Geometry: final body of the model. Coordinates: model frame, mm. Give positions to 0.01 mm unless a question says otherwise; leave off trailing zeros. Write each loop counter-clockwise with the first axis right and the second up, starting at its lowest first coordinate (ties: lowest second). Pieces come first, ordered by that corner, then holes.
from build123d import *

# Parameters (mm, degrees)
SPHERE001_ANGLE = 180
SPHERE_ANGLE    = 180


with BuildPart() as inner:
    # Sphere001 → Sphere001 (revolve)
    with BuildSketch(Plane.XZ):
        with BuildLine():
            ThreePointArc((0, -28), (28, 0), (0, 28))
            Line((0, 28), (0, -28))
        make_face()
    revolve(axis=Axis((0, 0, 0), (0, 0, 1)), revolution_arc=SPHERE001_ANGLE)


with BuildPart() as cut:
    # Sphere → Sphere (revolve)
    with BuildSketch(Plane.XZ):
        with BuildLine():
            ThreePointArc((0, -30), (30, 0), (0, 30))
            Line((0, 30), (0, -30))
        make_face()
    revolve(axis=Axis((0, 0, 0), (0, 0, 1)), revolution_arc=SPHERE_ANGLE)

    # Cut: cut Inner
    add(inner.part, mode=Mode.SUBTRACT)


solid = cut.part
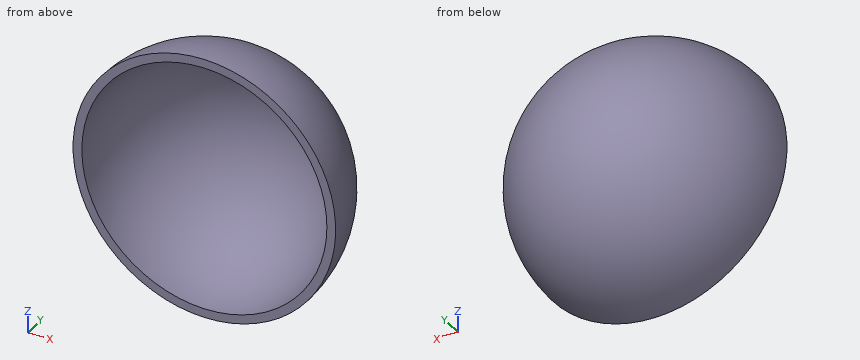
Q1. Section B-B on z = -1. Output: boundary loops of the cut face in (x, y).
Filled sheet:
outline: (-29.98, 0) - (-27.98, 0) arc R27.98 cw to (27.98, 0) - (29.98, 0) arc R29.98 ccw to start
Q2. Section C-C on x = 14. Output: boundary loops of the cut face in (y, z), plus the area to 3 significant figures.
Filled sheet:
outline: (0, -26.53) arc R26.53 ccw to (0, 26.53) - (0, 24.25) arc R24.25 cw to (0, -24.25) - close
area: 182 mm2
Q3. Pin query (flat end, axial travel): P1, Ø1.5, axis at x = 0, y = 8, coming from the -Z side; P2, Ø5, axis at x = -5, y = 25, coming from the +Z side; P3, Ø3, axis at y = 25.5, z = 1.5, coming from the +X side. Return the tip coordinate at first contact, or that it passes through.
Filled sheet:
P1: stops at z = -29.11
P2: stops at z = 19.27
P3: stops at x = 17.94
Q4. Ray query, line 1 along X through (y, z) = (10.5, -23); line 2 along Z through (x, y) = (12.5, 6.25); line 3 along X through (y, z) = (14.5, -8.5). Return the intervals inside material, ascending.
Filled sheet:
line 1: x = -16.15 to -12.03, 12.03 to 16.15
line 2: z = -26.55 to -24.26, 24.26 to 26.55
line 3: x = -24.85 to -22.39, 22.39 to 24.85
Q5. Section A-A on y = 16.25. Output: boundary loops of the cut face in (x, z), plus the area to 3 significant figures.
Filled sheet:
outline: circle Ø50.44 at (0, 0); hole circle Ø45.6 at (0, 0)
area: 364 mm2
